Answer from the drawing. Dimensions are ordinates in mm from the lowest x, y and z of the part. Give positions to 0.01 mm unless a question says otherwise; leave off trailing zeros. Order: outer loops, then holes, each group sorted by start corner. A loop starts at its lowest first (then second) coordinate and runs counter-clockwise, first axis right, second up. Notation, with made-up numbers: (42.5, 36.5) -> (90.5, 36.5) arc R23 cw to (90.5, 55.5) -> close; hole circle Ø6 at (82.5, -24). An arc over 180 degrees is marked (long way). Answer as a JSON object with one key per item and string values. Group by question number.
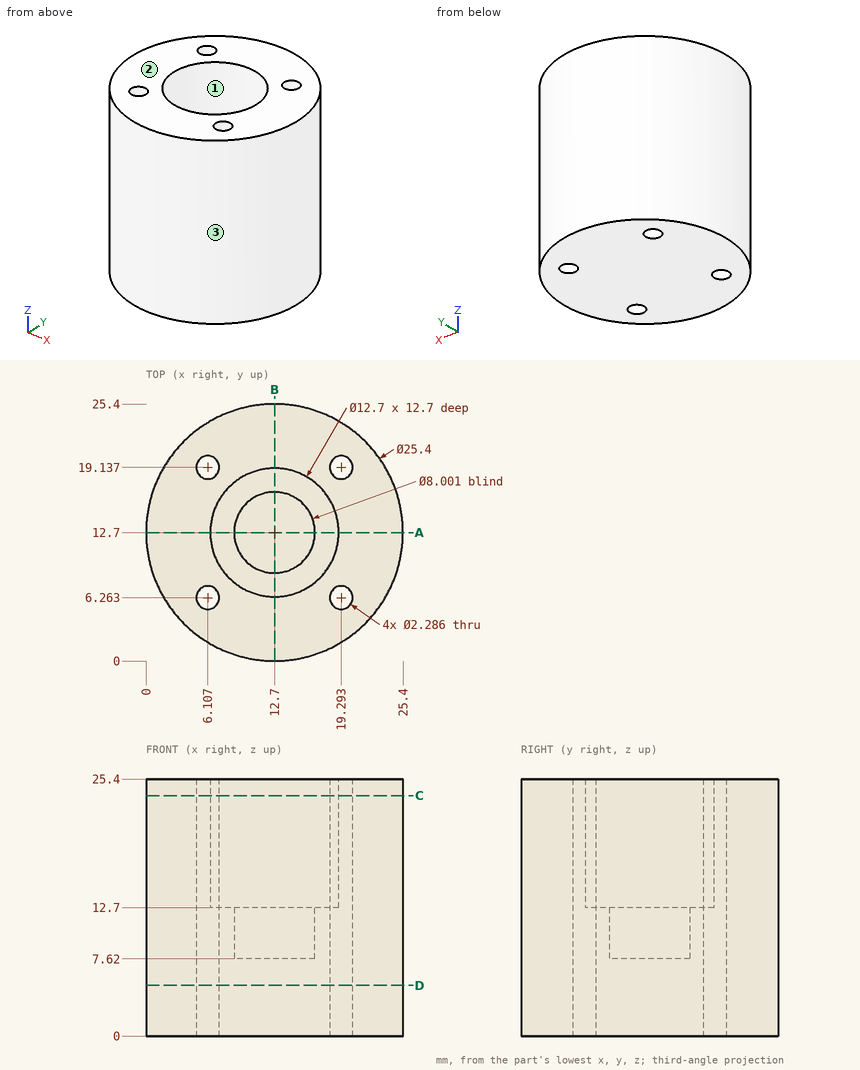
(1) Find the intervals of material crossed by line 1 along X through (y, z) = (20, 24.5) (1 decimal); line 2 along X through (y, z) = (12.75, 15.75); line 3 along Y through (x, z) = (19.25, 4.5) (1 decimal), in increasing order. Write a range as [from, to].
(2) A cutting plane is placed at C-C (z = 23.75). Determine the outline of the cut face in (x, y).
(3) A cutting plane is placed at D-D (z = 5). Determine the outline of the cut face in (x, y).
(4) Flat-ended cylindrical pins translate along their axes: pin 1 Ø1.8 at (x, y) = (6.11, 19.14) entering from +Z; pin 2 Ø10 at (x, z) = (20, 23) entering from +Y; pin 3 Ø9 at (x, y) = (11.5, 13) entering from +Z; pin 4 Ø4 at (x, z) = (4.5, 14) entering from +Y (1 decimal). Find the tip coordinate at first contact, or state that the pin passes through.
(5) For a pull along Y with two mould halves and no side action, classify the marked faces 1, 2 and 3 as +Y half, -Y half, draft (parallel to the pull), parting line (faces both ways), or undercut.
(6) A cutting plane is placed at A-A (y = 12.7). Determine the outline of the cut face in (x, z), and give its area (3 significant figures).
Check sheet entries:
{
 "1": {"line 1": "x = [2.3, 5.4], [6.9, 18.5], [20, 23.1]", "line 2": "x = [0, 6.35], [19.05, 25.4]", "line 3": "y = [1.8, 5.1], [7.4, 18], [20.3, 23.6]"},
 "2": {"outline": "circle Ø25.4 at (12.7, 12.7); hole circle Ø2.29 at (6.11, 6.26); hole circle Ø2.29 at (6.11, 19.14); hole circle Ø12.7 at (12.7, 12.7); hole circle Ø2.29 at (19.29, 6.26); hole circle Ø2.29 at (19.29, 19.14)"},
 "3": {"outline": "circle Ø25.4 at (12.7, 12.7); hole circle Ø2.29 at (6.11, 6.26); hole circle Ø2.29 at (6.11, 19.14); hole circle Ø2.29 at (19.29, 6.26); hole circle Ø2.29 at (19.29, 19.14)"},
 "4": {"pin 1": "passes through", "pin 2": "stops at y = 25.19", "pin 3": "stops at z = 12.7", "pin 4": "stops at y = 23.8"},
 "5": {"face 1": "undercut", "face 2": "draft", "face 3": "parting line"},
 "6": {"outline": "(0, 0) -> (25.4, 0) -> (25.4, 25.4) -> (19.05, 25.4) -> (19.05, 12.7) -> (16.7, 12.7) -> (16.7, 7.62) -> (8.7, 7.62) -> (8.7, 12.7) -> (6.35, 12.7) -> (6.35, 25.4) -> (0, 25.4) -> close", "area": "443 mm2"}
}
